Verification items for the finished model (mm, model axes). A direction names the side the tool comes from. Round coordinates to 2 decimals unless told otherwise and drop trailing zeros. Write each loop counter-clockwise with the first axis right and the second up, starting at its lowest first coordinate (ties: lowest second). Pieces come first, ordered by that corner, then holes. Notation, with made-up numbers: (-14, 87.25) - (11, 87.25) arc R21 cw to (11, 100.25) - close; hole circle Ø1 at (6, -20). An arc over 180 degrees is marked (long way). Answer as a JSON object with one key per item and string values. Group by question number.
1) Set-up check for faces 1 (the flat face through (-55, -8, 5.67)), 2 (the cylindrical face through (2, 16, 22)), 3 (the flat face through (-55, -8, 17.623)), 4 (the flat face through (-55, -12.086, 12)): record each of +Z, -Z, +X, -X, +Y, -Y from which the full face is reachable in a straight line by a thin tool's end or side.
2) Section check A-A (y = 3). Enter the section's corners in (x, z).
3) Go/stop test with flat-tipped pins: pin 1 Ø5 at (y, z) = (-3, 13) entering from -X; pin 2 Ø1 at (x, z) = (-55, 9.5) entering from -Y; pin 3 Ø2 at (x, y) = (-55.5, -7.5) entering from +Z. Record where each tip stops, or that it passes through.
4) Thickness scan on line 1 (X direction, y = 7.5, z = 9); line 2 (X direction, y = -11, z = 8); line 3 (Z direction, x = -17, y = -12.5). Record the ranges inside material, lowest first.
5) Mould release check, pull along Z, two halves, no side actions. Record for faces 5 (the cylindrical face through (-59.08, -8.134, 16.848)), 6 (the flat face through (-62, -8, 9)), 7 (the flat face through (-57, -8, 12)), 8 (the cylindrical face through (53.4, 0.17, 0.57)): +Z half, -Z half, draft (parallel to the pull), parting line (faces both ways), or undercut.
6) Section check B-B (x = 45). Enter the section's corners in (y, z).
```python
from build123d import *

# Parameters (mm, degrees)
SKETCH1_W           = 108
SKETCH1_H           = 34
BOSS_EXTRUDE1_DEPTH = 24
FILLET1_R           = 5
SKETCH2_W           = 11.95330434
SKETCH2_H           = 8.370070963
BOSS_EXTRUDE2_DEPTH = 3
SKETCH4_R           = 2.331694998
BOSS_EXTRUDE3_DEPTH = 8
FILLET2_R           = 0.5
CHAMFER1_SIZE       = 1
FILLET4_R           = 4
FILLET5_R           = 2


with BuildPart() as part:
    # Sketch1 → Boss-Extrude1 (new body)
    with BuildSketch(Plane.XY):
        Rectangle(SKETCH1_W, SKETCH1_H)
    extrude(amount=BOSS_EXTRUDE1_DEPTH)

    # Fillet1
    fillet1_edges = [part.edges().sort_by_distance(p)[0] for p in [
        (0, -17, 24),
        (0, -17, 0),
        (0, 17, 0),
        (0, 17, 24),
    ]]
    fillet(fillet1_edges, radius=FILLET1_R)

    # Sketch2 → Boss-Extrude2 (add)
    with BuildSketch(Plane.ZY.offset(54)):
        with Locations((11.64622902, -7.901268425)):
            Rectangle(SKETCH2_W, SKETCH2_H)
    extrude(amount=BOSS_EXTRUDE2_DEPTH)

    # Sketch4 → Boss-Extrude3 (add)
    with BuildSketch(Plane.ZY.offset(54)):
        with Locations(Location((14.518147435, -8.031501174, 0), (0, 0, 180))):
            Circle(SKETCH4_R)
        with Locations(Location((9.050368945, -8.031501174, 0), (0, 0, 180))):
            Circle(SKETCH4_R)
    extrude(amount=BOSS_EXTRUDE3_DEPTH)

    # Fillet2
    fillet2_edges = [part.edges().sort_by_distance(p)[0] for p in [
        (-62, -8.031501174, 16.849842433),
        (-62, -8.031501174, 11.382063944),
    ]]
    fillet(fillet2_edges, radius=FILLET2_R)

    # Chamfer1
    # the kernel refuses this chamfer: 1 mm, written as the material it takes off along each edge
    with BuildSketch(Plane(origin=(-57, -14.657986894, 17.62288119), x_dir=(-0.0274958766105891, 0, -0.9996219169112968), z_dir=(0, 1, 0))) as chamfer1_piece_1_section:
        Polygon((CHAMFER1_SIZE * 0.999621916911, -CHAMFER1_SIZE * 0.0274958766106), (-CHAMFER1_SIZE * 0.0274958766106, -CHAMFER1_SIZE * 0.999621916911), (0, 0), align=None)
    chamfer1_piece_1 = extrude(amount=13.513436938, mode=Mode.PRIVATE)
    chamfer1_piece_1 = chamfer1_piece_1 - Plane(origin=(-56.66854021, -8.031501174, 14.518147435), x_dir=(0, 0, -1), z_dir=(1, 0, 0)) * Cylinder(2.331694998, 32, mode=Mode.PRIVATE)
    add(chamfer1_piece_1, mode=Mode.SUBTRACT)
    with BuildSketch(Plane(origin=(-57, -3.716232943, 20.194564177), x_dir=(-0.02749587661058907, -0.9996219169112965, 0), z_dir=(0, 0, -1)), Plane(origin=(-57, -12.086303906, 3.097893862), x_dir=(-0.0274958766105891, 0.9996219169112968, 0), z_dir=(0, 0, 1))) as chamfer1_piece_2:
        Polygon((CHAMFER1_SIZE * 0.999621916911, -CHAMFER1_SIZE * 0.0274958766106), (-CHAMFER1_SIZE * 0.0274958766106, -CHAMFER1_SIZE * 0.999621916911), (0, 0), align=None)
    extrude(amount=17.096670315, mode=Mode.SUBTRACT)
    with BuildSketch(Plane(origin=(-57, -1.144549955, 5.66957685), x_dir=(-0.02749587661058907, 0, 0.9996219169112965), z_dir=(0, -1, 0))) as chamfer1_piece_3:
        Polygon((CHAMFER1_SIZE * 0.999621916911, -CHAMFER1_SIZE * 0.0274958766106), (-CHAMFER1_SIZE * 0.0274958766106, -CHAMFER1_SIZE * 0.999621916911), (0, 0), align=None)
    extrude(amount=13.513436938, mode=Mode.SUBTRACT)

    # Fillet4
    fillet4_edges = [part.edges().sort_by_distance(p)[0] for p in [
        (-54, 17, 12),
        (-54, 0, 0),
        (-54, -17, 12),
        (-54, 0, 24),
        (-54, -15.535533906, 22.535533906),
        (-54, -15.535533906, 1.464466094),
        (-54, 15.535533906, 22.535533906),
        (-54, 15.535533906, 1.464466094),
    ]]
    fillet(fillet4_edges, radius=FILLET4_R)

    # Fillet5
    fillet5_edges = [part.edges().sort_by_distance(p)[0] for p in [
        (54, 17, 12),
        (54, 0, 0),
        (54, 0, 24),
        (54, -17, 12),
        (54, -15.535533906, 22.535533906),
        (54, -15.535533906, 1.464466094),
        (54, 15.535533906, 22.535533906),
        (54, 15.535533906, 1.464466094),
    ]]
    fillet(fillet5_edges, radius=FILLET5_R)


solid = part.part
```
Returned:
{
 "1": {"face 1": "-Z, -X, +Y, -Y", "face 2": "+Z, +X, -X, +Y", "face 3": "+Z, -X, +Y, -Y", "face 4": "+Z, -Z, -X, -Y"},
 "2": {"outline": "(-54, 4) arc R4 ccw to (-50, 0) - (52, 0) arc R2 ccw to (54, 2) - (54, 22) arc R2 ccw to (52, 24) - (-50, 24) arc R4 ccw to (-54, 20) - close"},
 "3": {"pin 1": "x = -57", "pin 2": "y = -12.09", "pin 3": "z = 17.62"},
 "4": {"line 1": "-54 to 54", "line 2": "-57 to 54", "line 3": "0.03 to 23.97"},
 "5": {"face 5": "undercut", "face 6": "draft", "face 7": "undercut", "face 8": "-Z half"},
 "6": {"outline": "(-17, 5) arc R5 ccw to (-12, 0) - (12, 0) arc R5 ccw to (17, 5) - (17, 19) arc R5 ccw to (12, 24) - (-12, 24) arc R5 ccw to (-17, 19) - close"}
}
